Geometry: final body of the model. Coordinates: model frame, mm. A direction names the side the tool comes from. Round coordinates to 2 decimals unless told otherwise and drop trailing zeros. Loops run counter-clockwise (first coordinate to the right, second up) from the corner with the lowest first, then second, coordinate; pieces in that order, holes last. Notation, with made-up numbers: (19.25, 89.25) - (39.25, 89.25) arc R24 cw to (39.25, 122.25) - close; hole circle Ø2 at (57.5, 47.5). An arc over 180 degrees is marked (long way). Use CSV: the item, a comma, the result in double quotes.
from build123d import *

# Parameters (mm, degrees)
F1_DEPTH = 12.7
F2_W     = 31.75
F2_H     = 14.224
F3_DEPTH = 31.75
F4_R     = 6.35
F5_DEPTH = 25.4


with BuildPart() as f1:
    # F0 (on Front) → F1 (new body)
    with BuildSketch(Plane.XZ):
        Polygon((24.795182, 59.197172), (-6.954818, 59.197172), (-54.452818, 11.445172), (-54.452818, -10.652828), (72.293182, -10.652828), (72.293182, 11.445172), align=None)
    extrude(amount=F1_DEPTH)

    # F2 (on face) → F3 (join)
    with BuildSketch(Plane.XZ.offset(12.7)):
        with Locations((8.920182, 52.085172)):
            Rectangle(F2_W, F2_H)
        Polygon((-26.004818, 2.047172), (-26.004818, -10.652828), (43.845182, -10.652828), (43.845182, 2.047172), (24.795182, 21.097172), (-6.954818, 21.097172), align=None)
    extrude(amount=F3_DEPTH)

    # F4 (on face) → F5 (cut)
    with BuildSketch(Plane.XY.offset(59.197172)):
        with Locations((7.162185, -28.702)):
            Circle(F4_R)
    extrude(amount=-F5_DEPTH, mode=Mode.SUBTRACT)


solid = f1.part
Item 1: Section D-D on z = 48. Return the cut outline in (x, y), plus the area to 3 significant figures.
Final values:
outline,"(-18.09, -12.7) - (-6.95, -12.7) - (-6.95, -44.45) - (24.8, -44.45) - (24.8, -12.7) - (35.93, -12.7) - (35.93, 0) - (-18.09, 0) - close; hole circle Ø12.7 at (7.16, -28.7)"
area,"1,570 mm²"
Item 2: Material intervals for line 1 (Z direction, x = -4, y = -17); line 2 (X direction, y = -41, z = 45.5); line 3 (Y direction, x = 36, z = 33.5), sorted ascending.
Final values:
line 1,"z = -10.65 to 21.1, 44.97 to 59.2"
line 2,"x = -6.95 to 24.8"
line 3,"y = -12.7 to 0"
Item 3: Pin query (flat end, axial travel): P1, Ø11.5, axis at y = -32, z = 55, coming from the +X side; P2, Ø4.5, axis at y = -36.5, z = 51, coming from the -X side; P3, Ø10, axis at y = -27.5, z = -6.5, coming from the +X side. Return the tip coordinate at first contact, or that it passes through.
Final values:
P1,"stops at x = 24.8"
P2,"stops at x = -6.95"
P3,"stops at x = 43.85"
Item 4: Section C-C on y = -32. Return the cut outline in (x, z), plus the area to 3 significant figures.
Final values:
outline,"(-26, -10.65) - (43.85, -10.65) - (43.85, 2.05) - (24.8, 21.1) - (-6.95, 21.1) - (-26, 2.05) - close; (-6.95, 44.97) - (1.74, 44.97) - (1.74, 59.2) - (-6.95, 59.2) - close; (12.59, 44.97) - (24.8, 44.97) - (24.8, 59.2) - (12.59, 59.2) - close"
area,"2,150 mm²"
Item 5: Section B-B on z = -5. Return the cut outline in (x, y), plus the area to 3 significant figures.
Final values:
outline,"(-54.45, -12.7) - (-26, -12.7) - (-26, -44.45) - (43.85, -44.45) - (43.85, -12.7) - (72.29, -12.7) - (72.29, 0) - (-54.45, 0) - close"
area,"3,830 mm²"
Item 6: Section A-A on y = -20.5. Return the cut outline in (x, z).
Final values:
outline,"(-26, -10.65) - (43.85, -10.65) - (43.85, 2.05) - (24.8, 21.1) - (-6.95, 21.1) - (-26, 2.05) - close; (-6.95, 44.97) - (24.8, 44.97) - (24.8, 59.2) - (-6.95, 59.2) - close"
Item 7: Mould query, pull axis Y, two halves, no side actions, for faces 5 (the flat face through (8, 0, 17)), 6 (the flat face through (8, -44.45, 5)), 7 (the flat face through (43.845, -28, -4)), 8 (the cylindrical face through (6.336, -22.406, 52.185)). Classes: released by +Y, released by -Y, zero draft, split by the parting line, or undercut.
Final values:
face 5,"released by +Y"
face 6,"released by -Y"
face 7,"zero draft"
face 8,"undercut"
Item 8: Reachability of faces 1 (the flat face through (-26.005, -28, -4)), 2 (the flat face through (9, -28, 21.097)), 3 (the flat face through (-6.955, -28, 52)), 4 (the flat face through (24.795, -28, 52)) from +Z, -Z, +X, -X, +Y, -Y: full face, straight path, thin tool, end or side. Return the list, or none.
Final values:
face 1,"+Z, -Z, -X, -Y"
face 2,"+X, -X, -Y"
face 3,"+Z, -X, -Y"
face 4,"+Z, +X, -Y"
